Source: three-view drawing plus pictorial views. Frame: mm from the lowest corner of the part. Round coordinates to 2 decimals unless told otherwise and drop trailing zeros. Write each loop counter-clockwise with the first axis right and the second up, starting at its lowest first coordinate (ties: lowest second). Pieces come first, ordered by that corner, then holes. Notation, with made-up numbers: M 8,28 L 60,28 A16 ccw 60,41 Z; hole C -23,3 d6. An arc over 180 degrees is marked long. Answer in a Markdown table with one row per item.
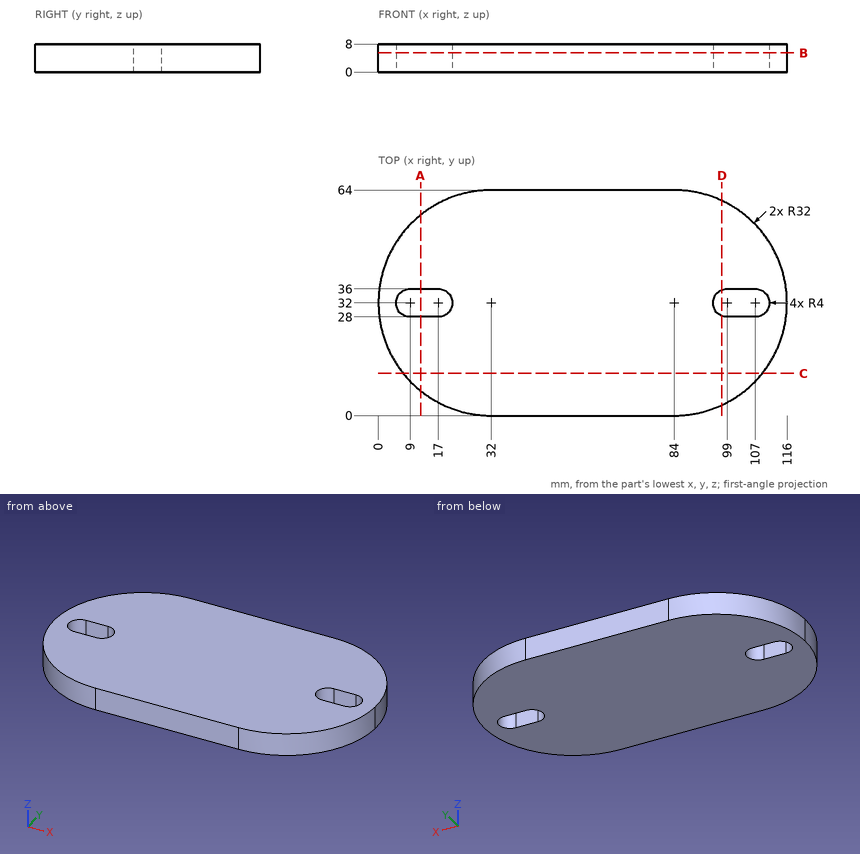
Q1. Material intervals for probe 1 along X at (y, z) = (29.5, 7.75); probe 2 along Y at (x, z) = (19, 5.5); probe 3 along Y at (x, z) = (97.5, 1.25), sorted ascending.
Solutions:
| item | result |
|---|---|
| probe 1 | x = 0.1 to 5.88, 20.12 to 95.88, 110.12 to 115.9 |
| probe 2 | y = 2.76 to 28.54, 35.46 to 61.24 |
| probe 3 | y = 2.99 to 28.29, 35.71 to 61.01 |
Q2. Section C-C (y = 12). Return loops of the section in (x, z), and give its area (3 significant figures).
Solutions:
| item | result |
|---|---|
| outline | M 7.02,0 L 108.98,0 L 108.98,8 L 7.02,8 Z |
| area | 816 mm2 |
Q3. Section D-D (x = 97.5). Return loops of the section in (y, z).
Solutions:
| item | result |
|---|---|
| outline | M 2.99,0 L 28.29,0 L 28.29,8 L 2.99,8 Z; M 35.71,0 L 61.01,0 L 61.01,8 L 35.71,8 Z |
Q4. Contact query for flat-ended pins moving along their axis: pin 1 Ø2 at (y, z) = (17, 2.5) entering from -X (3 decimals); pin 2 Ø2.5 at (x, z) = (13.5, 5.5) entering from -Y; pin 3 Ø4 at (x, z) = (19.5, 2.5) entering from +Y. Output: stop coordinate, or through.
Solutions:
| item | result |
|---|---|
| pin 1 | stops at x = 3.225 |
| pin 2 | stops at y = 5.05 |
| pin 3 | stops at y = 62.23 |
Q5. Section A-A (x = 12). Return loops of the section in (y, z).
Solutions:
| item | result |
|---|---|
| outline | M 7.02,0 L 28,0 L 28,8 L 7.02,8 Z; M 36,0 L 56.98,0 L 56.98,8 L 36,8 Z |
Q6. Section B-B (z = 5.5). Return loops of the section in (x, y).
Solutions:
| item | result |
|---|---|
| outline | M 32,0 L 84,0 A32 ccw 84,64 L 32,64 A32 ccw Z; hole M 9,28 L 17,28 A4 ccw 17,36 L 9,36 A4 ccw Z; hole M 99,28 L 107,28 A4 ccw 107,36 L 99,36 A4 ccw Z |
